Print and shaded views of the part. All mm, measured from the part's lowest x, y and z. A direction names the side the tool comes from. Give positions to 0.01 mm unless a question says otherwise; leave off trailing zeros. Loops run counter-clockwise (first coordinate to the right, second up) from the corner with the lowest first, then second, coordinate; pieces in that order, holes last.
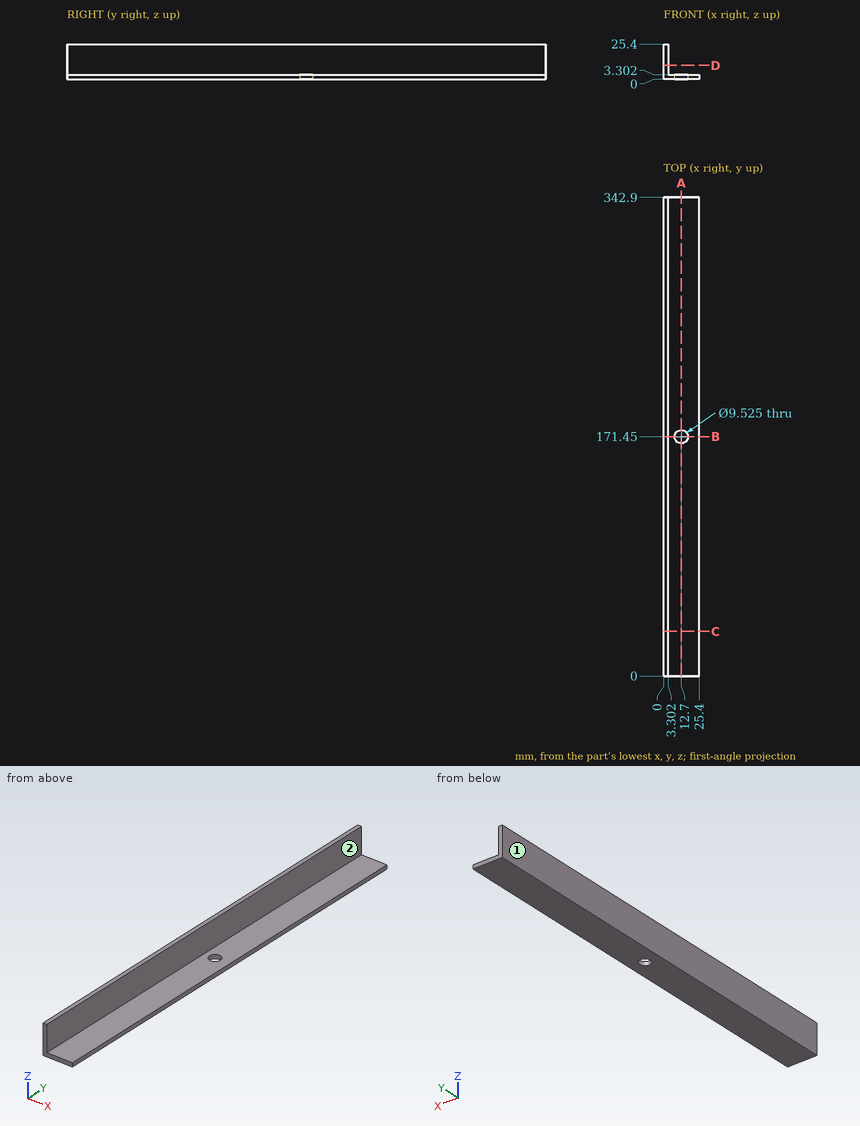
1. Saw through at A-A, the plane x = 12.7. List the corners of the cut face in (y, z).
Responses:
outline: (0, 0) - (166.69, 0) - (166.69, 3.3) - (0, 3.3) - close; (176.21, 0) - (342.9, 0) - (342.9, 3.3) - (176.21, 3.3) - close
2. Probe line 1 along Y through (x, z) = (12.7, 0.9); line 2 along Z through (x, y) = (6.25, 69.5). List the from-to ranges inside material, lowest first.
Responses:
line 1: y = 0 to 166.69, 176.21 to 342.9
line 2: z = 0 to 3.3
3. Saw through at D-D, the plane z = 10. List the corners of the cut face in (x, y), and give its area (3 significant figures).
Responses:
outline: (0, 0) - (3.3, 0) - (3.3, 342.9) - (0, 342.9) - close
area: 1,130 mm2
4. Drop flat-ended pins along their axis: pin 1 (5 mm diameter, centred on x = 15, y = 207, fed in from +Z); pin 2 (1.5 mm diameter, centred on y = 109.5, z = 8, fed in from +X); pin 3 (8.5 mm diameter, centred on x = 12.7, y = 171.45, fed in from +Z). Give the stop position or say it passes through.
Responses:
pin 1: stops at z = 3.3
pin 2: stops at x = 3.3
pin 3: passes through
5. Saw through at B-B, the plane y = 171.45. List the corners of the cut face in (x, z), and give its area (3 significant figures).
Responses:
outline: (0, 0) - (7.94, 0) - (7.94, 3.3) - (3.3, 3.3) - (3.3, 25.4) - (0, 25.4) - close; (17.46, 0) - (25.4, 0) - (25.4, 3.3) - (17.46, 3.3) - close
area: 125 mm2
6. Saw through at C-C, the plane y = 32. List the corners of the cut face in (x, z).
Responses:
outline: (0, 0) - (25.4, 0) - (25.4, 3.3) - (3.3, 3.3) - (3.3, 25.4) - (0, 25.4) - close
7. Tool access for the marked faces 1 and 2: list every direction of +Z, -Z, +X, -X, +Y, -Y with a clear straight run to the whole face (end or side of a thin tool).
Responses:
face 1: +Z, -Z, -X, +Y, -Y
face 2: +Z, +X, +Y, -Y
